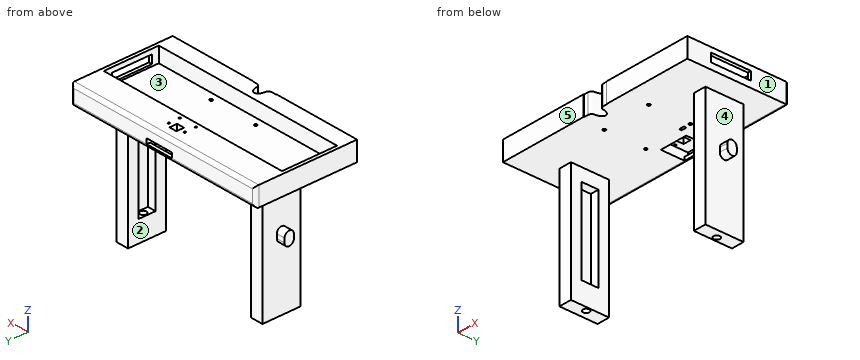
```python
from build123d import *

# Parameters (mm, degrees)
ESQUISSE1_W              = 240
ESQUISSE1_H              = 120
BOSS_EXTRU_1_DEPTH       = 23
ESQUISSE2_W              = 232
ESQUISSE2_H              = 65
ENL_V_MAT_EXTRU_1_DEPTH  = 18
CONG_1_R                 = 4
ESQUISSE7_R              = 1.75
ENL_V_MAT_EXTRU_3_DEPTH  = 10
ESQUISSE14_W             = 10
ESQUISSE14_H             = 47
ENL_V_MAT_EXTRU_9_DEPTH  = 43
ESQUISSE17_W             = 33
ESQUISSE17_H             = 6
ENL_V_MAT_EXTRU_11_DEPTH = 32
ESQUISSE18_W             = 33
ESQUISSE18_H             = 28
ENL_V_MAT_EXTRU_12_DEPTH = 7
ESQUISSE19_W             = 15
ESQUISSE19_H             = 45
BOSS_EXTRU_2_DEPTH       = 140
ESQUISSE20_W             = 100
ESQUISSE20_H             = 20
ENL_V_MAT_EXTRU_13_DEPTH = 10
ESQUISSE21_R             = 3.75
ENL_V_MAT_EXTRU_14_DEPTH = 40
ESQUISSE22_W             = 100
ESQUISSE22_H             = 20
ENL_V_MAT_EXTRU_15_DEPTH = 10
ESQUISSE23_R             = 3.75
ENL_V_MAT_EXTRU_16_DEPTH = 40
BOSS_EXTRU_3_DEPTH       = 10
BOSS_EXTRU_4_START       = 10
BOSS_EXTRU_4_DEPTH       = 10
ESQUISSE30_R             = 1.1
ESQUISSE30_W             = 9
ESQUISSE30_H             = 9
ENL_V_MAT_EXTRU_22_DEPTH = 30
ESQUISSE31_W             = 6
ESQUISSE31_H             = 3
ENL_V_MAT_EXTRU_23_DEPTH = 10
ENL_V_MAT_EXTRU_24_DEPTH = 40


with BuildPart() as part:
    # Esquisse1 → Boss.-Extru.1 (new body)
    with BuildSketch(Plane.XY):
        with Locations((-120, -60)):
            Rectangle(ESQUISSE1_W, ESQUISSE1_H)
    extrude(amount=BOSS_EXTRU_1_DEPTH)

    # Esquisse2 → Enlèv. mat.-Extru.1 (cut)
    with BuildSketch(Plane.XY.offset(23)):
        with Locations((-120, -67.5)):
            Rectangle(ESQUISSE2_W, ESQUISSE2_H)
    extrude(amount=-ENL_V_MAT_EXTRU_1_DEPTH, mode=Mode.SUBTRACT)

    # Congé1
    cong_1_edges = [part.edges().sort_by_distance(p)[0] for p in [
        (-120, 0, 0),
        (-240, 0, 11.5),
        (0, 0, 11.5),
        (-120, 0, 23),
    ]]
    fillet(cong_1_edges, radius=CONG_1_R)

    # Esquisse7 → Enlèv. mat.-Extru.3 (cut)
    with BuildSketch(Plane.XY.offset(5)):
        with Locations((-139.35, -42.66)):
            Circle(ESQUISSE7_R)
        with Locations((-139.35, -91.66)):
            Circle(ESQUISSE7_R)
        with Locations((-81.35, -91.66)):
            Circle(ESQUISSE7_R)
        with Locations((-81.35, -42.66)):
            Circle(ESQUISSE7_R)
    extrude(amount=-ENL_V_MAT_EXTRU_3_DEPTH, mode=Mode.SUBTRACT)

    # Esquisse14 → Enlèv. mat.-Extru.9 (cut)
    with BuildSketch(Plane.ZY.offset(4)):
        with Locations((12.363440201, -68.5)):
            Rectangle(ESQUISSE14_W, ESQUISSE14_H)
    extrude(amount=-ENL_V_MAT_EXTRU_9_DEPTH, mode=Mode.SUBTRACT)

    # Esquisse17 → Enlèv. mat.-Extru.11 (cut)
    with BuildSketch(Plane(origin=(0, 0, 0), x_dir=(1, 0, 0), z_dir=(0, 1, 0))):
        with Locations((-115, -7)):
            Rectangle(ESQUISSE17_W, ESQUISSE17_H)
    extrude(amount=-ENL_V_MAT_EXTRU_11_DEPTH, mode=Mode.SUBTRACT)

    # Esquisse18 → Enlèv. mat.-Extru.12 (cut)
    with BuildSketch(Plane(origin=(0, 0, 0), x_dir=(-1, 0, 0), z_dir=(0, 0, -1))):
        with Locations((115, -18)):
            Rectangle(ESQUISSE18_W, ESQUISSE18_H)
    extrude(amount=-ENL_V_MAT_EXTRU_12_DEPTH, mode=Mode.SUBTRACT)

    # Esquisse19 → Boss.-Extru.2 (add)
    with BuildSketch(Plane(origin=(0, 0, 0), x_dir=(-1, 0, 0), z_dir=(0, 0, -1))):
        with Locations((32.5, -53.5)):
            Rectangle(ESQUISSE19_W, ESQUISSE19_H)
        with Locations((207.5, -53.5)):
            Rectangle(ESQUISSE19_W, ESQUISSE19_H)
    extrude(amount=BOSS_EXTRU_2_DEPTH)

    # Esquisse20 → Enlèv. mat.-Extru.13 (cut)
    with BuildSketch(Plane.ZY.offset(40)):
        with Locations((-65, -53.5)):
            Rectangle(ESQUISSE20_W, ESQUISSE20_H)
    extrude(amount=-ENL_V_MAT_EXTRU_13_DEPTH, mode=Mode.SUBTRACT)

    # Esquisse21 → Enlèv. mat.-Extru.14 (cut)
    with BuildSketch(Plane.XY.offset(-115)):
        with Locations((-35, -53.5)):
            Circle(ESQUISSE21_R)
    extrude(amount=-ENL_V_MAT_EXTRU_14_DEPTH, mode=Mode.SUBTRACT)

    # Esquisse22 → Enlèv. mat.-Extru.15 (cut)
    with BuildSketch(Plane(origin=(-200, 0, 0), x_dir=(0, 0, -1), z_dir=(1, 0, 0))):
        with Locations((65, -53.5)):
            Rectangle(ESQUISSE22_W, ESQUISSE22_H)
    extrude(amount=-ENL_V_MAT_EXTRU_15_DEPTH, mode=Mode.SUBTRACT)

    # Esquisse23 → Enlèv. mat.-Extru.16 (cut)
    with BuildSketch(Plane.XY.offset(-115)):
        with Locations((-205, -53.5)):
            Circle(ESQUISSE23_R)
    extrude(amount=-ENL_V_MAT_EXTRU_16_DEPTH, mode=Mode.SUBTRACT)

    # Esquisse25 → Boss.-Extru.3 (add)
    with BuildSketch(Plane(origin=(-25, 0, 0), x_dir=(0, 0, -1), z_dir=(1, 0, 0))):
        with BuildLine():
            Line((55, -48), (60, -48))
            ThreePointArc((60, -48), (65.5, -53.5), (60, -59))
            Line((60, -59), (55, -59))
            ThreePointArc((55, -59), (49.5, -53.5), (55, -48))
        make_face()
    extrude(amount=BOSS_EXTRU_3_DEPTH)

    # Esquisse26 → Boss.-Extru.4 (add)
    with BuildSketch(Plane.ZY.offset(215).offset(BOSS_EXTRU_4_START)):
        with BuildLine():
            Line((-60, -48), (-55, -48))
            ThreePointArc((-55, -48), (-49.5, -53.5), (-55, -59))
            Line((-55, -59), (-60, -59))
            ThreePointArc((-60, -59), (-65.5, -53.5), (-60, -48))
        make_face()
    extrude(amount=-BOSS_EXTRU_4_DEPTH)

    # Esquisse30 → Enlèv. mat.-Extru.22 (cut)
    with BuildSketch(Plane(origin=(0, 0, 10), x_dir=(-1, 0, 0), z_dir=(0, 0, -1))):
        with Locations((108.5, -30)):
            Circle(ESQUISSE30_R)
        with Locations((129.5, -30)):
            Circle(ESQUISSE30_R)
        with Locations((129.5, -16.96)):
            Circle(ESQUISSE30_R)
        with Locations((108.5, -16.96)):
            Circle(ESQUISSE30_R)
        with Locations((118.79, -17.08)):
            Rectangle(ESQUISSE30_W, ESQUISSE30_H)
    extrude(amount=-ENL_V_MAT_EXTRU_22_DEPTH, mode=Mode.SUBTRACT)

    # Esquisse31 → Enlèv. mat.-Extru.23 (cut)
    with BuildSketch(Plane.XY.offset(5)):
        with Locations((-91.35, -42.5)):
            Rectangle(ESQUISSE31_W, ESQUISSE31_H)
    extrude(amount=-ENL_V_MAT_EXTRU_23_DEPTH, mode=Mode.SUBTRACT)

    # Esquisse32 → Enlèv. mat.-Extru.24 (cut)
    with BuildSketch(Plane.XY.offset(23)):
        with BuildLine():
            Line((-135, -119.5), (-135, -120))
            Line((-135, -120), (-105, -120))
            Line((-105, -120), (-105, -119.5))
            Line((-105, -119.5), (-110, -119.5))
            add(Edge.make_bspline(
                [(-130, -119.5), (-129.411520636, -119.5), (-125.206007881, -118.2698291), (-126.070515277, -112.049296748), (-119.869966777, -103.868703164), (-113.838690693, -112.386692695), (-114.398901471, -118.075641111), (-110.922134696, -119.5), (-110, -119.5)],
                knots=[0, 0, 0, 0, 0.144122834, 0.276784549, 0.509496521, 0.778688307, 0.880905797, 1, 1, 1, 1], degree=3))
            Line((-130, -119.5), (-135, -119.5))
        make_face()
    extrude(amount=-ENL_V_MAT_EXTRU_24_DEPTH, mode=Mode.SUBTRACT)


solid = part.part
```
Source: CAD feature listing. Evaluate the final solid. Frame: model axes, mm. Face numbers are marked on the shaded views. A direction names the side the tool comes from. Coordinates: 2 decimals unless noted, no trailing zeros. Loops run counter-clockwise (first coordinate to the right, second up) from the corner with the lowest first, then second, coordinate; pieces in that order, holes last. Notation, with made-up numbers: M -11,8.5 L 45,8.5 A19 cw 45,29.5 Z; hole C 60.25,78.5 d2. An arc over 180 degrees is marked long. Put each result on its own line as item: value. Start each with the question number.
1) Contact query for flat-ended pins moving along their axis: pin 1 Ø3 at (y, z) = (-28.5, -56) entering from -X; pin 2 Ø1 at (x, z) = (-36.5, -96.5) entering from +Y; pin 3 Ø5.5 at (x, z) = (-219.5, -58.5) entering from +Y; pin 4 Ø1.5 at (x, y) = (-152, -52.5) entering from +Z. Output: stop coordinate, or through.
2) Ray query, L1, parallel to X at y = -91.66, z = 2.7; L2, parallel to Z at x = -33, y = -59.5; L3, parallel to X at y = -56, z = -128.5. Return the intervals inside material, ascending. Write a range as from..to.
3) Cut plane B-B on x = -43. Return the cut outline in (y, z).
4) Pull-direction query (Y, two-part tool) for the marked faces 3, 4 and 5; classes: pulls with the +Y half, pulls with the -Y half, needs draft (parallel to the pull), parting line crosses it, or undercut.
5) Reachability of the marked faces 1 and 2 from +Z, -Z, +X, -X, +Y, -Y: full face, straight path, thin tool, end or side. Return the list, or none.
6) Cut plane A-A on z = -20.5. Return the cut outline in (x, y).
The answers:
1. pin 1: passes through
1. pin 2: stops at y = -31
1. pin 3: stops at y = -48
1. pin 4: stops at z = 5
2. L1: x = -240..-141.1, -137.6..-83.1, -79.6..0
2. L2: z = -140..-115, -15..5
2. L3: x = -215..-207.8, -202.2..-200, -40..-37.8, -32.2..-25
3. outline: M -120,0 L -4,0 A4 ccw 0,4 L 0,19 A4 ccw -4,23 L -35,23 L -35,5 L -100,5 L -100,23 L -120,23 Z
4. face 3: undercut
4. face 4: needs draft
4. face 5: pulls with the -Y half
5. face 1: +Z, -Z, +X, +Y, -Y
5. face 2: -Z, +Y, -Y
6. outline: M -215,-76 L -200,-76 L -200,-63.5 L -210,-63.5 L -210,-43.5 L -200,-43.5 L -200,-31 L -215,-31 Z; M -40,-76 L -25,-76 L -25,-31 L -40,-31 L -40,-43.5 L -30,-43.5 L -30,-63.5 L -40,-63.5 Z
